Work out the finished part from the listing and answer in its coordinate system (mm). A direction names the side the tool comes from. Round coordinates to 2 decimals unless told otherwise and drop trailing zeros. Loops run counter-clockwise (first coordinate to the right, second up) from the corner with the lowest first, then second, coordinate; pieces in that order, holes last. Notation, with made-up numbers: (23, 40.25) - (49, 40.25) arc R15 ccw to (49, 46.25) - close; hole circle Ø9 at (19.25, -30.75). An arc over 180 degrees is marked (long way). Return JSON: item names as keys, results as strings.
from build123d import *

# Parameters (mm, degrees)
F1_DEPTH = 7.5
F3_R     = 2.15
F4_DEPTH = 20
F2_R     = 2.15
F5_DEPTH = 20
F6_START = -2
F2_R_2   = 3.65
F6_DEPTH = 18
F7_START = -2
F3_R_2   = 3.65
F7_DEPTH = 18
F8_R     = 1


with BuildPart() as f1:
    # F0 (on Top) → F1 (new body, symmetric)
    with BuildSketch(Plane.XY):
        Polygon((0, 20), (0, 0), (20, 0), (20, 2), (2, 20), align=None)
    extrude(amount=F1_DEPTH, both=True)

    # F3 (on face) → F4 (cut)
    with BuildSketch(Plane.XZ):
        with Locations((10, 0)):
            Circle(F3_R)
    extrude(amount=-F4_DEPTH, mode=Mode.SUBTRACT)

    # F2 (on face) → F5 (cut)
    with BuildSketch(Plane(origin=(0, 0, 0), x_dir=(0, -1, 0), z_dir=(-1, 0, 0))):
        with Locations((-10, 0)):
            Circle(F2_R)
    extrude(amount=-F5_DEPTH, mode=Mode.SUBTRACT)

    # F2 (on face) → F6 (cut)
    with BuildSketch(Plane(origin=(0, 0, 0), x_dir=(0, -1, 0), z_dir=(-1, 0, 0)).offset(F6_START)):
        with Locations((-10, 0)):
            Circle(F2_R_2)
        with Locations((-10, 0)):
            Circle(F2_R, mode=Mode.SUBTRACT)
    extrude(amount=-F6_DEPTH, mode=Mode.SUBTRACT)

    # F3 (on face) → F7 (cut)
    with BuildSketch(Plane.XZ.offset(F7_START)):
        with Locations((10, 0)):
            Circle(F3_R_2)
        with Locations((10, 0)):
            Circle(F3_R, mode=Mode.SUBTRACT)
    extrude(amount=-F7_DEPTH, mode=Mode.SUBTRACT)

    # F8
    f8_edges = [f1.edges().sort_by_distance(p)[0] for p in [
        (0, 0, 0),
        (20, 0, 0),
        (20, 2, 0),
        (2, 20, 0),
        (0, 20, 0),
    ]]
    fillet(f8_edges, radius=F8_R)


solid = f1.part
1) Flat-ended cylindrical pins translate along their axes: pin 1 (6 mm diameter, centred on y = 10, z = 0.5, fed in from +X); pin 2 (6.5 mm diameter, centred on x = 10, z = 0, fed in from +Y); pin 3 (7 mm diameter, centred on x = 10, z = 0, fed in from -Y); pin 4 (5 mm diameter, centred on y = 7, z = 4, fed in from +X). Find the tip coordinate at first contact, or state that the pin passes through.
Verdict:
{"pin 1": "stops at x = 2", "pin 2": "stops at y = 2", "pin 3": "stops at y = 0", "pin 4": "stops at x = 17.5"}
2) Section D-D (x = 11.5) is taken. Give the vertices of the cut face in (y, z), and give its area (3 significant figures).
Verdict:
{"outline": "(0, -7.5) - (10.5, -7.5) - (10.5, -3.62) arc R3.65 cw to (8.5, -3.33) - (2, -3.33) - (2, -1.54) - (0, -1.54) - close; (0, 1.54) - (2, 1.54) - (2, 3.33) - (8.5, 3.33) arc R3.65 cw to (10.5, 3.62) - (10.5, 7.5) - (0, 7.5) - close", "area": "93.8 mm2"}
3) Section C-C (y = 4.25) is taken. Give the vertices of the cut face in (x, z), and give its area (3 significant figures).
Verdict:
{"outline": "(0, -7.5) - (17.75, -7.5) - (17.75, 7.5) - (0, 7.5) - close; hole circle Ø7.3 at (10, 0)", "area": "224 mm2"}
4) Section A-A (z = 0) is taken. Give the vertices of the cut face in (x, y), and give its area (3 significant figures).
Verdict:
{"outline": "(0, 1) arc R1 ccw to (1, 0) - (7.85, 0) - (7.85, 2) - (6.35, 2) - (6.35, 6.35) - (2, 6.35) - (2, 7.85) - (0, 7.85) - close; (0, 12.15) - (2, 12.15) - (2, 13.65) - (6.35, 13.65) - (6.35, 15.65) - (2.29, 19.71) arc R1 ccw to (1.59, 20) - (1, 20) arc R1 ccw to (0, 19) - close; (12.15, 0) - (19, 0) arc R1 ccw to (20, 1) - (20, 1.59) arc R1 ccw to (19.71, 2.29) - (15.65, 6.35) - (13.65, 6.35) - (13.65, 2) - (12.15, 2) - close", "area": "113 mm2"}
5) Section B-B (x = 4.75) is taken. Give the vertices of the cut face in (y, z), and give its area (3 significant figures).
Verdict:
{"outline": "(0, -7.5) - (17.25, -7.5) - (17.25, 7.5) - (0, 7.5) - close; hole circle Ø7.3 at (10, 0)", "area": "217 mm2"}
6) A tool of negligible diameter and unlimited length cuts with its end or side. For faces 1 (the cylindrical face through (13.86, 6.38, 0.47)), 2 (the cylindrical face through (7.85, 0.99, 0.09)), 3 (the cylindrical face through (6.38, 13.96, -0.47)), from which of +Z, -Z, +X, -X, +Y, -Y can it reach the whole face along a straight path? Write none if from no direction.
Verdict:
{"face 1": "+X", "face 2": "+Y, -Y", "face 3": "+Y"}
7) Determine the mould class of faces 4 (the cylindrical face through (5.06, 12.69, 2.47)), 5 (the flat face through (8, 8, 7.5)), 6 (the flat face through (12, 2, -2)), 7 (the flat face through (12, 0, 2)) for opening direction Z: pulls with the +Z half, pulls with the -Z half, needs draft (parallel to the pull), parting line crosses it, or undercut.
Verdict:
{"face 4": "undercut", "face 5": "pulls with the +Z half", "face 6": "undercut", "face 7": "needs draft"}
8) Find the intervals of material crossed by L1, parallel to Z at x = 10, y = 4.75; L2, parallel to X at y = 10.75, z = -2.25; L3, parallel to X at y = 3.75, z = -2, in increasing order.
Verdict:
{"L1": "z = -7.5 to -3.65, 3.65 to 7.5", "L2": "x = 0 to 2", "L3": "x = 0 to 6.95, 13.05 to 18.25"}
